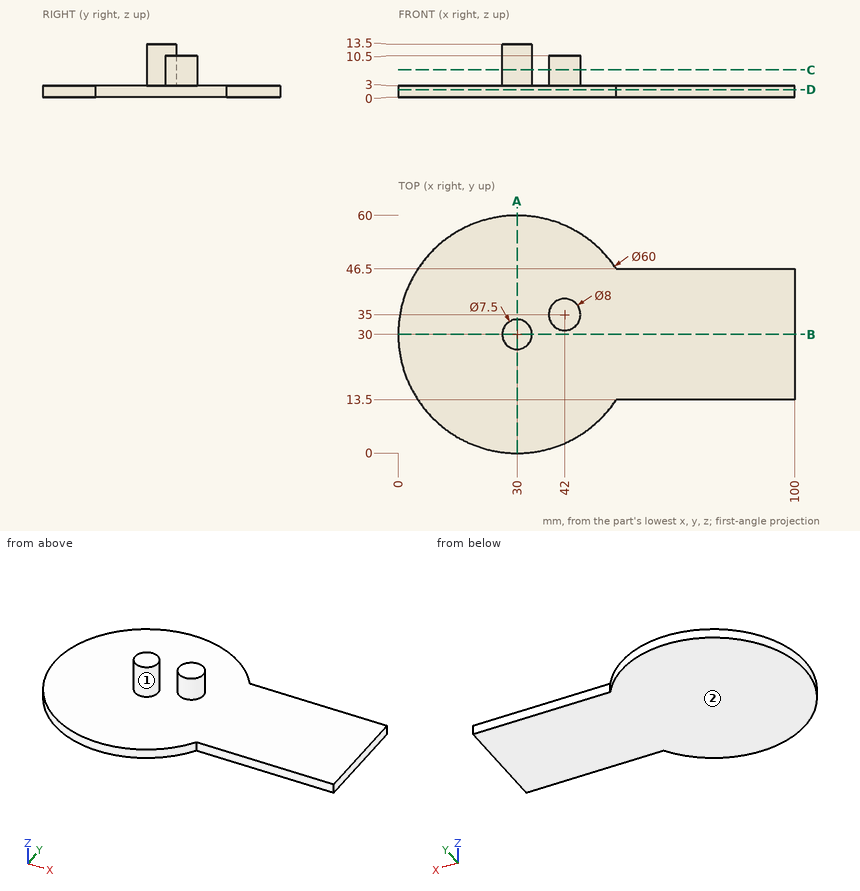
Design review of the part shown in the three views and the two pictorial views. Dimensions are in mm from the part's minimum x, y and z. Round coordinates to 2 decimals unless told otherwise and drop trailing zeros. Write each loop counter-clockwise with the first axis right and the second up, starting at its lowest first coordinate (ties: lowest second). Pieces come first, ordered by that corner, then holes.
Item 1: We need section A-A on x = 30. Write out the cut boundary in (y, z), and give its area (3 significant figures).
Item 2: The part is to be moulded in two halves that separate along X. For the marked faces 1 and 2, say which applies: +X half, -X half, draft (parallel to the pull), parting line (faces both ways), or undercut.
Item 3: We need section D-D on z = 2. Write out the cut boundary in (x, y), and give its area (3 significant figures).
Item 4: Clearance check with flat-ended pins moving along their axes: pin 1 Ø1.5 at (x, z) = (27.5, 2.5) entering from -Y; pin 2 Ø4 at (x, y) = (42, 34) entering from +Z; pin 3 Ø2.5 at (x, z) = (88.5, 1.5) entering from -Y. State where each tip first meets the part, or that it passes through.
Item 5: We need section B-B on y = 30. Write out the cut boundary in (x, z), and give its area (3 significant figures).
Item 6: We need section C-C on z = 7. Write out the cut boundary in (x, y).
Item 7: For probe 1 along Z at (x, y) = (85, 37); probe 2 along X at (y, z) = (27.5, 1); probe 3 along X at (y, z) = (42, 1), list the stretches that pass through material, from the lowest coordinate up.
Returned:
1. outline: (0, 0) - (60, 0) - (60, 3) - (33.75, 3) - (33.75, 13.5) - (26.25, 13.5) - (26.25, 3) - (0, 3) - close
1. area: 259 mm2
2. face 1: undercut
2. face 2: draft
3. outline: (55.05, 13.5) - (100, 13.5) - (100, 46.5) - (55.05, 46.5) arc R30 ccw (long way) to start
3. area: 4,200 mm2
4. pin 1: stops at y = 0.05
4. pin 2: stops at z = 10.5
4. pin 3: stops at y = 13.5
5. outline: (0, 0) - (100, 0) - (100, 3) - (33.75, 3) - (33.75, 13.5) - (26.25, 13.5) - (26.25, 3) - (0, 3) - close
5. area: 379 mm2
6. outline: circle Ø7.5 at (30, 30); circle Ø8 at (42, 35)
7. probe 1: z = 0 to 3
7. probe 2: x = 0.1 to 100
7. probe 3: x = 2.5 to 100
